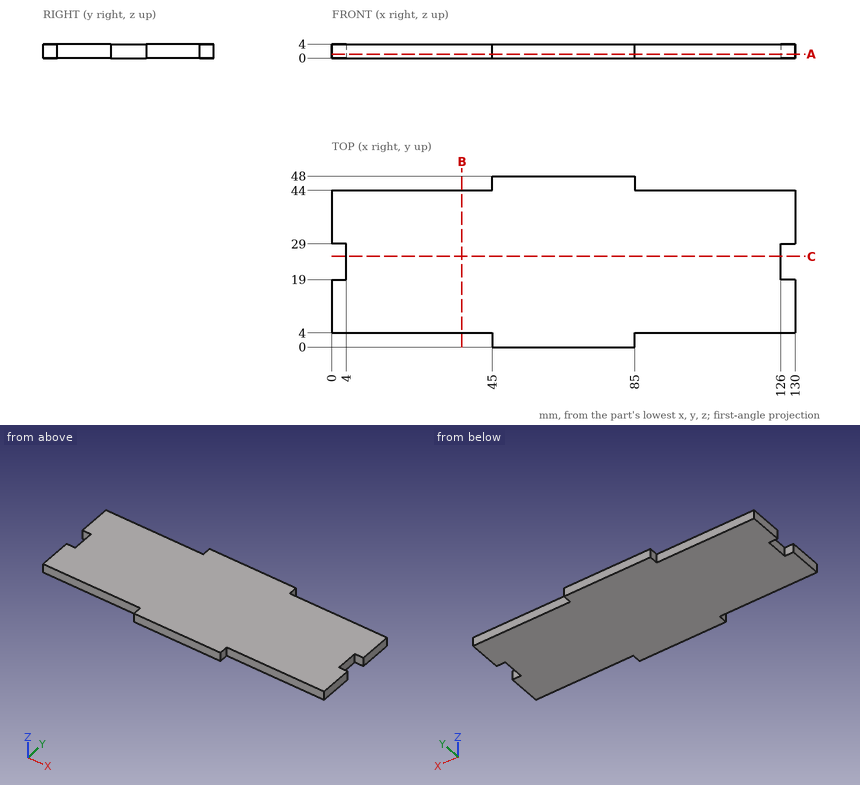
Drawing for the job (mm, zero at the part's lowest x, y, z). Give positions to 0.01 mm unless a question says otherwise; leave off trailing zeros. Write each loop counter-clockwise with the first axis right and the second up, starting at its lowest first coordinate (ties: lowest second). Pieces come first, ordered by that corner, then holes. Notation, with made-up numbers: (42, 74.5) - (75, 74.5) arc R27 cw to (75, 107.5) - close; hole circle Ø10 at (-19, -25.5). An arc over 180 degrees is marked (long way). Answer as CSV lines item,"result".
Q1. Drill centre lines: line 1 (X direction, y = 26, z = 3.5); line 2 (Y direction, x = 12.5, z = 3.35). Where is each one in solid material? Low to high. Write a range as from..to.
Result set:
line 1,"4..126"
line 2,"4..44"
Q2. Band-saw the part on C-C (y = 25.5). Give the cut face in (x, z).
Result set:
outline,"(4, 0) - (126, 0) - (126, 4) - (4, 4) - close"
Q3. Band-saw the part on A-A (z = 1.15). Give the cut face in (x, y).
Result set:
outline,"(0, 4) - (45, 4) - (45, 0) - (85, 0) - (85, 4) - (130, 4) - (130, 19) - (126, 19) - (126, 29) - (130, 29) - (130, 44) - (85, 44) - (85, 48) - (45, 48) - (45, 44) - (0, 44) - (0, 29) - (4, 29) - (4, 19) - (0, 19) - close"
Q4. Flat gauge pins, fed straight in: pin 1 Ø1.2 at (x, z) = (24, 1.5) entering from +Y; pin 2 Ø2 at (y, z) = (47, 1.5) entering from -X; pin 3 Ø1.2 at (y, z) = (45.5, 2) entering from +X. Where does each tip first touch, or does it go through?
Result set:
pin 1,"y = 44"
pin 2,"x = 45"
pin 3,"x = 85"
Q5. Band-saw the part on B-B (x = 36.5). Give the cut face in (y, z), and give its area (3 significant figures).
Result set:
outline,"(4, 0) - (44, 0) - (44, 4) - (4, 4) - close"
area,"160 mm²"
